```python
from build123d import *

# Parameters (mm, degrees)
BOSS_EXTRUDE1_DEPTH = 2
BOSS_EXTRUDE2_DEPTH = 1
SKETCH3_R           = 0.5
CUT_EXTRUDE1_DEPTH  = 64.683462008
CIRPATTERN1_COUNT   = 3


with BuildPart() as part:
    # Sketch1 → Boss-Extrude1 (new body)
    with BuildSketch(Plane.XY):
        Polygon((0, 34.063665882), (-29.5, -17.031832941), (29.5, -17.031832941), align=None)
    extrude(amount=BOSS_EXTRUDE1_DEPTH)

    # Sketch2 → Boss-Extrude2 (add, symmetric)
    with BuildSketch(Plane(origin=(0, 0, 0), x_dir=(0, 0, -1), z_dir=(1, 0, 0))):
        Polygon((-2, -0.936334118), (-2, -5.031832941), (-17, -5.031832941), (-17, -8.146867769), (-24.319391415, -5.376586618), (-25.381329824, -8.182346196), (-47, 0), (-47, 2.259927745), (-5, 32.063665882), (-2, 32.063665882), (-2, 24.063665882), (-5, 24.063665882), (-5, -0.936334118), align=None)
    extrude(amount=BOSS_EXTRUDE2_DEPTH, both=True)

    # Sketch3 → Cut-Extrude1 (cut, through all)
    with BuildSketch(Plane.XY.offset(2)):
        with Locations((-8, -14.531832941)):
            Circle(SKETCH3_R)
        with Locations(Location((8, -14.531832941, 0), (0, 0, 180))):
            Circle(SKETCH3_R)
    cut_extrude1 = extrude(amount=-CUT_EXTRUDE1_DEPTH, mode=Mode.SUBTRACT)

    # CirPattern1: Cut-Extrude1 ×3 about axis
    cirpattern1_axis = Axis((0, 0, 0), (0, 0, 1))
    for i in range(1, CIRPATTERN1_COUNT):
        add(cut_extrude1.rotate(cirpattern1_axis, i * 360 / CIRPATTERN1_COUNT), mode=Mode.SUBTRACT)


solid = part.part
```
Geometry check sheet. Reference: the model listing, model coordinates, mm. A direction names the side the tool comes from. Coordinates: 2 decimals unless noted, no trailing zeros. Write each loop counter-clockwise with the first axis right and the second up, starting at its lowest first coordinate (ties: lowest second). Pieces come first, ordered by that corner, then holes. Notation, with made-up numbers: M 75.25,-38 L 79.25,-38 A22 ccw 79.25,-17 Z; hole C 49,23.25 d6. An arc over 180 degrees is marked long. One line per item, written item: value. Start each with the question number.
(1) Sectioned sample at C-C, the plane z = 35.5. Enter the section's corners in (x, y).
(2) Tool access check on faces 4 (the face through (0, -7, 17)), 5 (the face through (0, 32.064, 4)), 6 (the face through (0, 12, 5)). Record the directions out of +Z, -Z, +X, -X, +Y, -Y that give a thin tool (end or side, any length) a straight path to the whole face; none if there is none.
(3) Sectioned sample at D-D, the plane x = 22.5. Enter the section's corners in (y, z), and give its area (3 significant figures).
(4) Sectioned sample at A-A, the plane y = 21. Enter the section's corners in (x, z).
(5) Scan lines: line 1 along Z through (x, y) = (-1.5, 20); line 2 along X through (y, z) = (-3, 33.5); line 3 along Y through (x, z) = (-8, 1.35). Record each from-to range of solid material in increasing order. Write a range as [from, to].
(6) Release check for a two-part mould opening along Y. For faces 1 (the face through (0, -0.936, 4)), 2 (the face through (0, -5.032, 9)), 3 (the face through (-1, 8, 19)) record: released by +Y, released by -Y, zero draft, split by the parting line, or undercut.
(7) Depth check by flat-ended pin: pin 1 (10 mm diameter, centred on x = -6.5, y = 23, fed in from +Z); pin 2 (1.6 mm diameter, centred on x = 0.5, z = 3.5, fed in from +Y); pin 3 (0.6 mm diameter, centred on x = 0, y = -7, fed in from -Z); pin 4 (2 mm diameter, centred on x = 0, z = 8, fed in from -Y). Enter the tip coordinate at first touch or a pass-through.
(8) Sectioned sample at B-B, the plane y = 30. Enter the section's corners in (x, z).
Filled sheet:
1. outline: M -1,-4.35 L 1,-4.35 L 1,10.42 L -1,10.42 Z
2. face 4: +X, -X, -Y
2. face 5: +Z, +X, -X, +Y
2. face 6: +X, -X
3. outline: M -17.03,0 L -4.91,0 L -4.91,2 L -17.03,2 Z
3. area: 24.2 mm²
4. outline: M -7.54,0 L 7.54,0 L 7.54,2 L -7.54,2 Z; M -1,5 L 1,5 L 1,20.59 L -1,20.59 Z
5. line 1: [0, 2]
5. line 2: [-1, 1]
5. line 3: [-17.03, -15.03], [-14.03, 20.21]
6. face 1: undercut
6. face 2: released by -Y
6. face 3: zero draft
7. pin 1: z = 2
7. pin 2: y = 32.06
7. pin 3: z = 0
7. pin 4: y = -5.03
8. outline: M -2.35,0 L 2.35,0 L 2.35,2 L 1,2 L 1,7.91 L -1,7.91 L -1,2 L -2.35,2 Z
